The model under review builds one solid part; all positions refer to its coordinate system, in mm. Coordinates: 2 decimals unless noted, no trailing zeros. Loops run counter-clockwise (first coordinate to the right, second up) from the corner with the lowest first, then second, coordinate; pieces in that order, holes last. Notation, with made-up numbers: (52.25, -24) - (83.25, -24) arc R23 cw to (83.25, -16) - close; hole circle Ø9 at (-39, 86). An arc over 180 degrees is marked (long way). Answer in a Markdown table with one row per item. Add a question column.
(1) For P1, Ø8, axis at x = 12, z = 15.5, coming from the +Y side; P2, Ø10, axis at x = 6.5, z = 15.5, coming from the -Y side; P3, Ø2, axis at x = 11.5, z = 6, coming from the -Y side, all flat-tipped, find the tip position at first contact; note any pin that passes through.
(2) We need section D-D on y = -24. Write out the cut boundary in (x, z), plus the area to 3 significant figures.
(3) We need section C-C on y = -5. Write out the cut boundary in (x, z), plus the area to 3 significant figures.
(4) We need section A-A on z = 9.5. Write out the cut boundary in (x, y).
(5) We need section B-B on x = 0. Write out the cut boundary in (y, z), plus the area to 3 significant figures.
(6) Mouldability with a two-part tool opening along Z and no side actions: class faces 1 (the cylindrical face through (0.224, -28.994, 9.786)), 2 (the cylindrical face through (0.224, -31.998, 9.709)), 3 (the flat face through (-16, -13, 10)), 4 (the flat face through (0, -16, 0)) as +Z half, -Z half, draft (parallel to the pull), parting line (faces both ways), or undercut.
(7) For line 1 along Y through (x, z) = (0, 9.75); line 2 along Z through (x, y) = (-6.5, -22.5); line 3 along Y through (x, z) = (8.5, 8.5), list the stretches that pass through material, from the lowest coordinate up.
from build123d import *

# Parameters (mm, degrees)
F0_R     = 16
F1_DEPTH = 19
F3_DEPTH = 16
F4_R     = 13
F5_DEPTH = 25
F6_R     = 6.5
F7_DEPTH = 32.001


with BuildPart() as f1:
    # F0 (on Top) → F1 (new body)
    with BuildSketch(Plane.XY):
        Circle(F0_R)
    extrude(amount=F1_DEPTH)

    # F2 (on Right) → F3 (join, symmetric)
    with BuildSketch(Plane.YZ):
        with BuildLine():
            Line((0, 19), (-22.5, 19))
            ThreePointArc((-22.5, 19), (-32, 9.5), (-22.5, 0))
            Line((-22.5, 0), (0, 0))
            Line((0, 0), (0, 19))
        make_face()
    extrude(amount=F3_DEPTH, both=True)

    # F4 (on face) → F5 (cut)
    with BuildSketch(Plane.XY.offset(19)):
        Circle(F4_R)
    extrude(amount=-F5_DEPTH, mode=Mode.SUBTRACT)

    # F6 (on face) → F7 (cut, through all)
    with BuildSketch(Plane.YZ.offset(16)):
        with Locations((-22.5, 9.5)):
            Circle(F6_R)
    extrude(amount=-F7_DEPTH, mode=Mode.SUBTRACT)


solid = f1.part
Outcome:
| question | item | result |
|---|---|---|
| 1 | P1 | y = 13.86 |
| 1 | P2 | y = -31.95 |
| 1 | P3 | y = -31.67 |
| 2 | outline | (-16, 0.12) - (16, 0.12) - (16, 3.18) - (-16, 3.18) - close; (-16, 15.82) - (16, 15.82) - (16, 18.88) - (-16, 18.88) - close |
| 2 | area | 196 mm² |
| 3 | outline | (-16, 0) - (-12, 0) - (-12, 19) - (-16, 19) - close; (12, 0) - (16, 0) - (16, 19) - (12, 19) - close |
| 3 | area | 152 mm² |
| 4 | outline | (-16, -32) - (16, -32) - (16, -29) - (-16, -29) - close; (-16, -16) - (16, -16) - (16, 0) arc R16 ccw to (-16, 0) - close; hole circle Ø26 at (0, 0) |
| 5 | outline | (-22.5, 0) - (-13, 0) - (-13, 19) - (-22.5, 19) arc R9.5 ccw to start; (13, 0) - (16, 0) - (16, 19) - (13, 19) - close; hole circle Ø13 at (-22.5, 9.5) |
| 5 | area | 247 mm² |
| 6 | face 1 | undercut |
| 6 | face 2 | parting line |
| 6 | face 3 | draft |
| 6 | face 4 | -Z half |
| 7 | line 1 | -32 to -29, -16 to -13, 13 to 16 |
| 7 | line 2 | 0 to 3, 16 to 19 |
| 7 | line 3 | -31.95 to -28.92, -16.08 to -9.84, 9.84 to 13.56 |
